Design review of the part built by this model. Coordinates are the model's own, in mm. Face numbers are marked on the shaded views. A direction names the side the tool comes from. Coordinates: 2 decimals unless noted, no trailing zeros. Loops run counter-clockwise (first coordinate to the right, second up) from the corner with the lowest first, then second, coordinate; pieces in that order, holes last. Notation, with made-up numbers: (78, 71.25) -> (121, 71.25) arc R24 ccw to (121, 104.25) -> close; hole circle Ø2 at (56, 71.5). An arc over 180 degrees is marked (long way). Use one line per item in the form item = value. Start each with the question number.
1. Consider section A-A (z = 0). State the section outline as (x, y) points, then the cut area to 3 significant figures.
2. Wall thickness on line 1 (X direction, y = 1.6, z = 0); line 2 (Z direction, x = 0, y = 12.15); line 3 (Y direction, x = 74.5, z = 8.5): over which ranges is each line inside the solid? List them lowest first. Write a range as from..to.
3. Consider section D-D (z = -6). State the section outline as (x, y) points, then the cut area to 3 significant figures.
4. Consider section C-C (y = 12.75). State the section outline as (x, z) points.
5. Consider section B-B (x = -1). State the section outline as (y, z) points, then the cut area to 3 significant figures.
6. For pin 1 (1.5 mm diameter, centred on y = 7.5, z = -6, fed in from +X); pin 2 (5 mm diameter, centred on y = 3.5, z = 3, fed in from -X); pin 3 (6.5 mm diameter, centred on x = 0, z = 0, fed in from -Y), all flat-tipped, find the tip position at first contact; note any pin that passes through.
7. Machinability: for the marked faces 1, 2 and 3, which of the approach directions +Z, -Z, +X, -X, +Y, -Y give a long, thin tool a straight path to every point of the face, cutting with its end or side? Answer none if there is none.
from build123d import *

# Parameters (mm, degrees)
SKETCH_2_R          = 2
SKETCH_2_R_2        = 4
EXTRUDE_1_DEPTH     = 15
SKETCH_3_W          = 98.28308004
SKETCH_3_H          = 42.939209726
CUT_EXTRUDE_1_DEPTH = 10
SKETCH_4_W          = 17.609413282
SKETCH_4_H          = 10.32275951
EXTRUDE_2_DEPTH     = 15
SKETCH_5_W          = 36.098979715
SKETCH_5_H          = 26.284001105
CUT_EXTRUDE_2_DEPTH = 10


with BuildPart() as part:
    # 草图2 → 凸台-拉伸1 (new body)
    with BuildSketch(Plane(origin=(0, 0, 0), x_dir=(1, 0, 0), z_dir=(0, 1, 0))):
        with BuildLine():
            Line((0, 10), (100, 10))
            ThreePointArc((100, 10), (110, 0), (100, -10))
            Line((100, -10), (0, -10))
            ThreePointArc((0, -10), (-10, 0), (0, 10))
        make_face()
        with Locations(Location((0, 0, 0), (0, 0, 270))):
            Circle(SKETCH_2_R, mode=Mode.SUBTRACT)
        with Locations(Location((10.16682634, 0, 0), (0, 0, 270))):
            Circle(SKETCH_2_R, mode=Mode.SUBTRACT)
        with Locations(Location((20.833686735, 0, 0), (0, 0, 270))):
            Circle(SKETCH_2_R, mode=Mode.SUBTRACT)
        with Locations(Location((32.412244599, 0, 0), (0, 0, 270))):
            Circle(SKETCH_2_R, mode=Mode.SUBTRACT)
        with Locations(Location((100, 0, 0), (0, 0, 270))):
            Circle(SKETCH_2_R, mode=Mode.SUBTRACT)
        with Locations(Location((88.357359208, 0, 0), (0, 0, 270))):
            Circle(SKETCH_2_R_2, mode=Mode.SUBTRACT)
        with Locations(Location((73.321402027, 0, 0), (0, 0, 270))):
            Circle(SKETCH_2_R_2, mode=Mode.SUBTRACT)
    extrude(amount=EXTRUDE_1_DEPTH)

    # 草图3 → 切除-拉伸1 (cut)
    with BuildSketch(Plane(origin=(0, 15, 0), x_dir=(1, 0, 0), z_dir=(0, 1, 0))):
        with Locations((75.503288201, -4.727650364)):
            Rectangle(SKETCH_3_W, SKETCH_3_H)
    extrude(amount=-CUT_EXTRUDE_1_DEPTH, mode=Mode.SUBTRACT)

    # 草图4 → 凸台-拉伸2 (add)
    with BuildSketch(Plane(origin=(0, 15, 0), x_dir=(1, 0, 0), z_dir=(0, 1, 0))):
        with Locations((15.041411071, 0.216864696)):
            Rectangle(SKETCH_4_W, SKETCH_4_H)
    extrude(amount=-EXTRUDE_2_DEPTH)

    # 草图5 → 切除-拉伸2 (cut)
    with BuildSketch(Plane.XZ):
        with Locations((2.252741217, 0.303610574)):
            Rectangle(SKETCH_5_W, SKETCH_5_H)
    extrude(amount=-CUT_EXTRUDE_2_DEPTH, mode=Mode.SUBTRACT)


solid = part.part
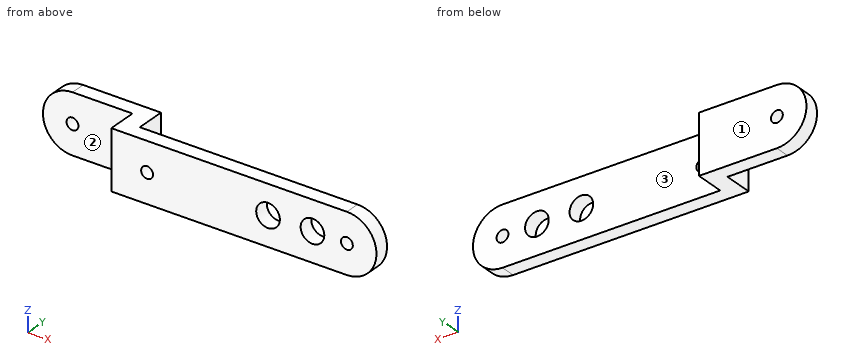
Geometry check:
q1.outline = (-10, 10) -> (-2, 10) -> (-2, 15) -> (-10, 15) -> close; (2, 10) -> (20.3, 10) -> (20.3, 0) -> (30.41, 0) -> (30.41, 5) -> (26.36, 5) -> (26.36, 15) -> (2, 15) -> close; (34.41, 0) -> (69.32, 0) -> (69.32, 5) -> (34.41, 5) -> close; (77.32, 0) -> (84.36, 0) -> (84.36, 5) -> (77.32, 5) -> close; (92.36, 0) -> (98, 0) -> (98, 5) -> (92.36, 5) -> close; (102, 0) -> (110, 0) -> (110, 5) -> (102, 5) -> close
q1.area = 521 mm²
q2.line_1 = 20.3..30.41, 34.41..69.32, 77.32..84.36, 92.36..98, 102..110
q2.line_2 = -10..-2, 2..10
q2.line_3 = 0..5
q3.outline = (-8, 10) -> (20.3, 10) -> (20.3, 0) -> (108, 0) -> (108, 5) -> (26.36, 5) -> (26.36, 15) -> (-8, 15) -> close
q3.area = 641 mm²
q4.outline = (0, -10) -> (26.36, -10) -> (26.36, 10) -> (0, 10) arc R10 ccw to start; hole circle Ø4 at (0, 0)
q5.outline = (10, -9.95) -> (15, -9.95) -> (15, -1.73) -> (10, -1.73) -> close; (10, 1.73) -> (15, 1.73) -> (15, 9.95) -> (10, 9.95) -> close
q5.area = 82.2 mm²
q6.pin_1 = 26.36
q6.pin_2 = 20.3
q6.pin_3 = 10
q7.face_1 = +Z, -Z, +X, -X, +Y
q7.face_2 = +Z, -Z, -X, -Y
q7.face_3 = +Z, -Z, +X, +Y
